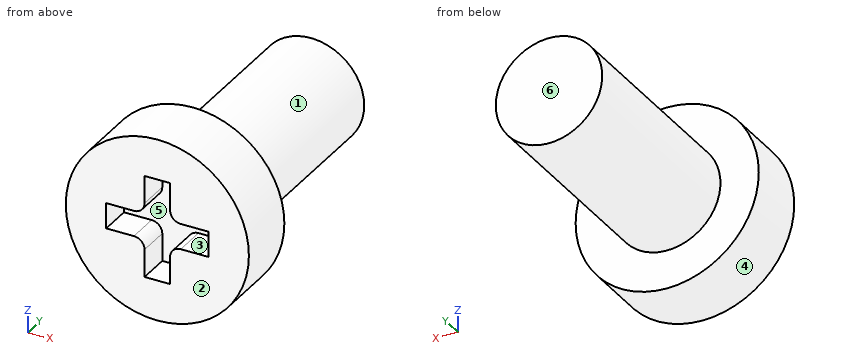
from build123d import *

# Parameters (mm, degrees)
SKETCH_1_R          = 4.3
EXTRUDE_1_DEPTH     = 3
SKETCH_2_R          = 2.5
EXTRUDE_2_DEPTH     = 10
CUT_EXTRUDE_1_DEPTH = 1.5


with BuildPart() as part:
    # 草图1 → 凸台-拉伸1 (new body)
    with BuildSketch(Plane(origin=(0, 0, 0), x_dir=(1, 0, 0), z_dir=(0, 1, 0))):
        Circle(SKETCH_1_R)
    extrude(amount=EXTRUDE_1_DEPTH)

    # 草图2 → 凸台-拉伸2 (add)
    with BuildSketch(Plane(origin=(0, 3, 0), x_dir=(1, 0, 0), z_dir=(0, 1, 0))):
        Circle(SKETCH_2_R)
    extrude(amount=EXTRUDE_2_DEPTH)

    # 草图3 → 切除-拉伸1 (cut)
    with BuildSketch(Plane.XZ):
        with BuildLine():
            Line((-0.6, 1.1), (-0.6, 2.4))
            Line((-0.6, 2.4), (0.6, 2.4))
            Line((0.6, 2.4), (0.6, 1.1))
            ThreePointArc((0.6, 1.1), (0.746446609, 0.746446609), (1.1, 0.6))
            Line((1.1, 0.6), (2.4, 0.6))
            Line((2.4, 0.6), (2.4, -0.6))
            Line((2.4, -0.6), (1.1, -0.6))
            ThreePointArc((1.1, -0.6), (0.746446609, -0.746446609), (0.6, -1.1))
            Line((0.6, -1.1), (0.6, -2.4))
            Line((0.6, -2.4), (-0.6, -2.4))
            Line((-0.6, -2.4), (-0.6, -1.1))
            ThreePointArc((-0.6, -1.1), (-0.746446609, -0.746446609), (-1.1, -0.6))
            Line((-1.1, -0.6), (-2.4, -0.6))
            Line((-2.4, -0.6), (-2.4, 0.6))
            Line((-2.4, 0.6), (-1.1, 0.6))
            ThreePointArc((-1.1, 0.6), (-0.746446609, 0.746446609), (-0.6, 1.1))
        make_face()
    extrude(amount=-CUT_EXTRUDE_1_DEPTH, mode=Mode.SUBTRACT)


solid = part.part
Work out the finished part from the listing and answer in its coordinate system (mm). Face numbers are marked on the shaded views. A direction names the side the tool comes from. Round coordinates to 2 decimals unless told otherwise and drop trailing zeros. Write each loop counter-clockwise with the first axis right and the second up, starting at its lowest first coordinate (ties: lowest second). Pieces come first, ordered by that corner, then holes. Notation, with made-up numbers: (-21.75, -29.5) -> (4.25, -29.5) arc R18 cw to (4.25, 3.5) -> close; hole circle Ø7 at (21, 80.25). An arc over 180 degrees is marked (long way). Write each question's results on one line, items separated by ' | '.
Item 1: Which of the six approach directions +Z, -Z, +X, -X, +Y, -Y give full straight-line access (tool end or side, diameter ignored) to the marked faces 1, 2 and 3?
Result set:
face 1: +Y | face 2: +Z, -Z, +X, -X, -Y | face 3: -Y
Item 2: The mould has two halves that part along Z. Classify the marked faces 4, 5 and 6: +Z half, -Z half, draft (parallel to the pull), parting line (faces both ways), or undercut.
Result set:
face 4: parting line | face 5: undercut | face 6: draft
Item 3: Flat-ended cylindrical pins translate along their axes: P1, Ø1, axis at x = 0, y = 11, coming from the +Z side; P2, Ø0.6, axis at y = 1, z = -1.5, coming from the +X side; P3, Ø0.6, axis at x = 1.5, y = 1, coming from the -Z side; P4, Ø3, axis at x = 1.5, y = 1.5, coming from the -Z side. Find the tip coordinate at first contact, or state that the pin passes through.
Result set:
P1: z = 2.5 | P2: x = 4.13 | P3: z = -4.13 | P4: z = -4.3
Item 4: A cutting plane is placed at D-D, the plane y = 7.5. Determine the outline of the cut face in (x, z).
Result set:
outline: circle Ø5 at (0, 0)
Item 5: A cutting plane is placed at A-A, the plane y = 1. Determine the outline of the cut face in (x, z), plus the area to 3 significant figures.
Result set:
outline: circle Ø8.6 at (0, 0); hole (-2.4, -0.6) -> (-1.1, -0.6) arc R0.5 cw to (-0.6, -1.1) -> (-0.6, -2.4) -> (0.6, -2.4) -> (0.6, -1.1) arc R0.5 cw to (1.1, -0.6) -> (2.4, -0.6) -> (2.4, 0.6) -> (1.1, 0.6) arc R0.5 cw to (0.6, 1.1) -> (0.6, 2.4) -> (-0.6, 2.4) -> (-0.6, 1.1) arc R0.5 cw to (-1.1, 0.6) -> (-2.4, 0.6) -> close | area: 47.8 mm^2
Item 6: A cutting plane is placed at C-C, the plane z = 0. Determine the outline of the cut face in (x, y).
Result set:
outline: (-4.3, 0) -> (-2.4, 0) -> (-2.4, 1.5) -> (2.4, 1.5) -> (2.4, 0) -> (4.3, 0) -> (4.3, 3) -> (2.5, 3) -> (2.5, 13) -> (-2.5, 13) -> (-2.5, 3) -> (-4.3, 3) -> close
Item 7: A cutting plane is placed at B-B, the plane x = 0. Determine the outline of the cut face in (y, z), plus the area to 3 significant figures.
Result set:
outline: (0, -4.3) -> (3, -4.3) -> (3, -2.5) -> (13, -2.5) -> (13, 2.5) -> (3, 2.5) -> (3, 4.3) -> (0, 4.3) -> (0, 2.4) -> (1.5, 2.4) -> (1.5, -2.4) -> (0, -2.4) -> close | area: 68.6 mm^2
Item 8: Find the intervals of material crossed by line 1 along Y through (x, z) = (2.75, -0.5); line 2 along Y through (x, z) = (1.75, 0.5); line 3 along X through (y, z) = (1.5, 3.5), in increasing order. Write a range as [from, to].
Result set:
line 1: [0, 3] | line 2: [1.5, 13] | line 3: [-2.5, 2.5]
